Verification items for this drawing (mm, ordinates from the low corner). Round coordinates to 2 decimals unless told otherwise and drop trailing zeros. Order: outer loops, then holes, each group sorted by start corner. A loop starts at its lowest first (then second) coordinate and runs counter-clockwise, first axis right, second up. Notation, with made-up numbers: (44.5, -26) - (60.5, -26) arc R14 ccw to (60.5, -18) - close; hole circle Ø2 at (-24.5, 40.5). An arc over 180 degrees is marked (long way). Use a Markdown table: item, result. Add a question column.
(1) Thickness scan on line 1 along X through (y, z) = (2.85, 86.5); line 2 along Z through (x, y) = (26.5, 2.5). Record the ranges inside material, lowest first. Write a range as [from, to].
(2) Gauge pin test, flat ends, axial feed: P1, Ø2.5, axis at y = 1.5, z = 104, coming from the +X side; P2, Ø2.5, axis at x = 151, y = 2, coming from the +Z side; P3, Ø2.5, axis at y = 2.5, z = 104, coming from the -X side. Record the tip position at first contact, or that the pin passes through.
(3) Section check A-A on x = 149.5. Record the boundary of the cut face in (y, z).
(4) Section check B-B on z = 19. Record the boundary of the cut face in (x, y).
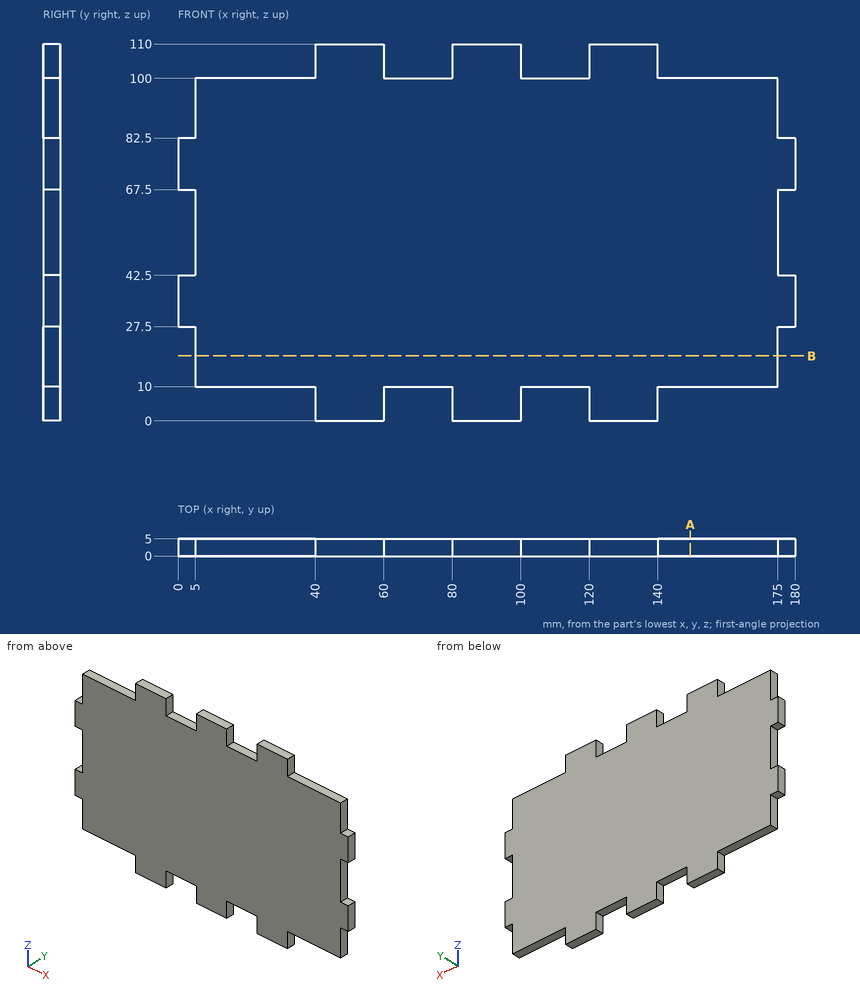
Check sheet entries:
| question | item | result |
|---|---|---|
| 1 | line 1 | x = [5, 175] |
| 1 | line 2 | z = [10, 100] |
| 2 | P1 | stops at x = 140 |
| 2 | P2 | stops at z = 100 |
| 2 | P3 | stops at x = 40 |
| 3 | outline | (0, 10) - (5, 10) - (5, 100) - (0, 100) - close |
| 4 | outline | (5, 0) - (175, 0) - (175, 5) - (5, 5) - close |
